```python
from build123d import *

# Parameters (mm, degrees)
F0_W     = 100
F0_H     = 12
F0_R     = 4
F1_DEPTH = 5
F2_R     = 2
F3_SIZE  = 0.6


with BuildPart() as f1:
    # F0 (on Top) → F1 (new body)
    with BuildSketch(Plane.XY):
        with Locations((25, 0)):
            Rectangle(F0_W, F0_H)
        with Locations((-19, 0)):
            Circle(F0_R, mode=Mode.SUBTRACT)
        with BuildLine():
            Line((69, -4), (0, -4))
            ThreePointArc((0, -4), (-4, 0), (0, 4))
            Line((0, 4), (69, 4))
            ThreePointArc((69, 4), (73, 0), (69, -4))
        make_face(mode=Mode.SUBTRACT)
    extrude(amount=F1_DEPTH)

    # F2
    f2_edges = [f1.edges().sort_by_distance(p)[0] for p in [
        (-25, -6, 2.5),
        (-25, 6, 2.5),
        (75, 6, 2.5),
        (75, -6, 2.5),
    ]]
    fillet(f2_edges, radius=F2_R)

    # F3
    f3_edges = [f1.edges().sort_by_distance(p)[0] for p in [
        (25, 6, 0),
        (74.414214, 5.414214, 0),
        (-24.414214, 5.414214, 0),
        (75, 0, 0),
        (-25, 0, 0),
        (74.414214, -5.414214, 0),
        (-24.414214, -5.414214, 0),
        (25, -6, 0),
        (-23, 0, 0),
        (34.5, 4, 0),
        (73, 0, 0),
        (34.5, -4, 0),
        (-4, 0, 0),
    ]]
    chamfer(f3_edges, length=F3_SIZE)


solid = f1.part
```
The listing builds one solid part. Answer for the finished solid, in the listing's coordinates (mm). A direction names the side the tool comes from. Give positions to 0.01 mm unless a question says otherwise; leave off trailing zeros. Write each loop counter-clockwise with the first axis right and the second up, starting at its lowest first coordinate (ties: lowest second). Pieces come first, ordered by that corner, then holes. Notation, with made-up numbers: (74.5, 56.5) -> (108.5, 56.5) arc R30 cw to (108.5, 91.5) -> close; hole circle Ø10 at (11, 52). An arc over 180 degrees is marked (long way). Write item = value, one per line. Start each with the question number.
1) Straight lines are drawn through the part: line 1 along Y through (x, z) = (-19, 1.9); line 2 along X through (y, z) = (2.25, 0.65); line 3 along X through (y, z) = (2.75, 3.5). For each, find the intervals that lie inside material, in ascending order.
2) Determine the mould class of faces 4 (the face through (24, -6, 3)), 5 (the face through (-4.2, -0.1, 0.4)), 6 (the face through (-25, 0, 3)), 7 (the face through (-24.43, 5.4, 2.83)) for opening direction Y: +Y half, -Y half, draft (parallel to the pull), parting line (faces both ways), or undercut.
3) The part is cut by section A-A, the plane y = 0. Determine the outline of the cut face in (x, z).
4) Which of the six approach directions +Z, -Z, +X, -X, +Y, -Y give full straight-line access (tool end or side, diameter ignored) to faces 1 (the face through (34, 4, 3)), 2 (the face through (73.2, 0.1, 0.4)), 3 (the face through (74.4, 5.43, 2.83))?
5) The part is cut by section B-B, the plane z = 2.45. Determine the outline of the cut face in (x, y).
6) The part is cut by section C-C, the plane x = -19. Determine the outline of the cut face in (y, z).
7) Each of these flat-tipped pins is pushed along its axis until it touches: pin 1 (7 mm diameter, centred on x = -19, y = 0, fed in from -Z); pin 2 (2 mm diameter, centred on x = 4, z = 0.5, fed in from -Y). Where does it stop, or does it pass through?
Solutions:
q1.line_1 = -6 to -4, 4 to 6
q1.line_2 = -25 to -22.31, -15.69 to -3.31, 72.31 to 75
q1.line_3 = -25 to -21.9, -16.1 to -2.9, 71.9 to 75
q2.face_4 = -Y half
q2.face_5 = undercut
q2.face_6 = draft
q2.face_7 = +Y half
q3.outline = (-25, 0.6) -> (-24.4, 0) -> (-23.6, 0) -> (-23, 0.6) -> (-23, 5) -> (-25, 5) -> close; (-15, 0.6) -> (-14.4, 0) -> (-4.6, 0) -> (-4, 0.6) -> (-4, 5) -> (-15, 5) -> close; (73, 0.6) -> (73.6, 0) -> (74.4, 0) -> (75, 0.6) -> (75, 5) -> (73, 5) -> close
q4.face_1 = +Z, -Z
q4.face_2 = -Z
q4.face_3 = +Z, -Z, +X, +Y
q5.outline = (-25, -4) arc R2 ccw to (-23, -6) -> (73, -6) arc R2 ccw to (75, -4) -> (75, 4) arc R2 ccw to (73, 6) -> (-23, 6) arc R2 ccw to (-25, 4) -> close; hole circle Ø8 at (-19, 0); hole (0, -4) -> (69, -4) arc R4 ccw to (69, 4) -> (0, 4) arc R4 ccw to start
q6.outline = (-6, 0.6) -> (-5.4, 0) -> (-4.6, 0) -> (-4, 0.6) -> (-4, 5) -> (-6, 5) -> close; (4, 0.6) -> (4.6, 0) -> (5.4, 0) -> (6, 0.6) -> (6, 5) -> (4, 5) -> close
q7.pin_1 = through
q7.pin_2 = -6
